from build123d import *

# Parameters (mm, degrees)
SKETCH1_R           = 4
BOSS_EXTRUDE1_DEPTH = 300
SKETCH2_R           = 3
BOSS_EXTRUDE2_DEPTH = 10
SKETCH3_R           = 1
CUT_EXTRUDE1_DEPTH  = 3
SKETCH4_R           = 4
SKETCH4_R_2         = 3
CUT_EXTRUDE2_DEPTH  = 10
SKETCH5_R           = 1
CUT_EXTRUDE3_DEPTH  = 3


with BuildPart() as part:
    # Sketch1 → Boss-Extrude1 (new body)
    with BuildSketch(Plane.XY):
        Circle(SKETCH1_R)
    extrude(amount=BOSS_EXTRUDE1_DEPTH)

    # Sketch2 → Boss-Extrude2 (add)
    with BuildSketch(Plane.XY.offset(300)):
        Circle(SKETCH2_R)
    extrude(amount=BOSS_EXTRUDE2_DEPTH)

    # Sketch3 → Cut-Extrude1 (cut, symmetric)
    with BuildSketch(Plane(origin=(0, 0, 0), x_dir=(1, 0, 0), z_dir=(0, 1, 0))):
        with Locations((0, -305)):
            Circle(SKETCH3_R)
    extrude(amount=CUT_EXTRUDE1_DEPTH, both=True, mode=Mode.SUBTRACT)

    # Sketch4 → Cut-Extrude2 (cut)
    with BuildSketch(Plane(origin=(0, 0, 0), x_dir=(-1, 0, 0), z_dir=(0, 0, -1))):
        Circle(SKETCH4_R)
        Circle(SKETCH4_R_2, mode=Mode.SUBTRACT)
    extrude(amount=-CUT_EXTRUDE2_DEPTH, mode=Mode.SUBTRACT)

    # Sketch5 → Cut-Extrude3 (cut, symmetric)
    with BuildSketch(Plane(origin=(0, 0, 0), x_dir=(1, 0, 0), z_dir=(0, 1, 0))):
        with Locations((0, -5)):
            Circle(SKETCH5_R)
    extrude(amount=CUT_EXTRUDE3_DEPTH, both=True, mode=Mode.SUBTRACT)


solid = part.part
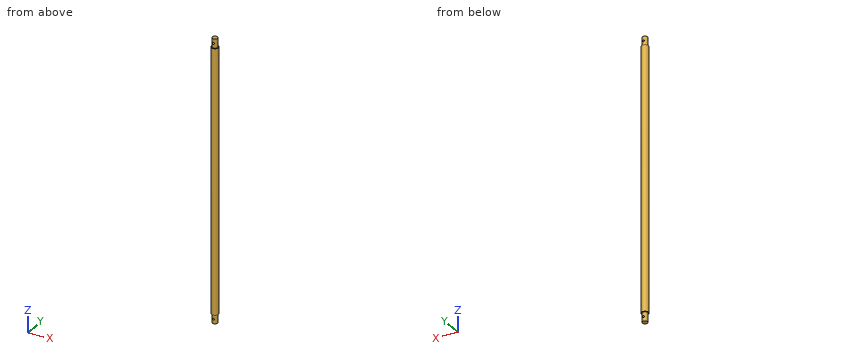
Design review of the part built by this model. Coordinates are the model's own, in mm. Round coordinates to 2 decimals unless told otherwise and drop trailing zeros. Order: outer loops, then holes, each group sorted by start corner. A loop starts at its lowest first (then second) coordinate and runs counter-clockwise, first axis right, second up. Notation, with made-up numbers: M -7,5.25 L 3,5.25 A25 ccw 3,35.25 Z; hole C 73.25,52 d2. An arc over 180 degrees is marked long. Answer as CSV lines item,"result". Start each with the question number.
1) Add section A-A (y = 0). Give the boundary of the cut face in (x, z).
2) For pin 1 Ø1.5 at (x, y) = (0, 1) entering from -Z; pin 2 Ø2.5 at (x, z) = (0, 5) entering from -Y; pin 3 Ø1 at (y, z) = (-2.5, 47.5) entering from -X, all flat-tipped, find the tip position at first contact; note any pin that passes through.
3) Wall thickness on line 1 along Z through (x, y) = (0, 0.5); line 2 along X through (y, z) = (2, 5); line 3 along Z through (x, y) = (2.5, -3): over which ranges is each line inside the solid? List them lowest first. Write a range as [from, to].
4) Add section B-B (z = 245). Give the boundary of the cut face in (x, y), then the cut area to 3 significant figures.
Resolved:
1,outline,"M -4,10 L -3,10 L -3,0 L 3,0 L 3,10 L 4,10 L 4,300 L 3,300 L 3,310 L -3,310 L -3,300 L -4,300 Z; hole C 0,5 d2; hole C 0,305 d2"
2,pin 1,"z = 0"
2,pin 2,"y = -3"
2,pin 3,"x = -3.46"
3,line 1,"[0, 4], [6, 304], [306, 310]"
3,line 2,"[-2.24, -1], [1, 2.24]"
3,line 3,"[10, 300]"
4,outline,"C 0,0 d8"
4,area,"50.3 mm^2"
